```python
from build123d import *

# Parameters (mm, degrees)
PAD002_DEPTH   = 40
SKETCH006_R    = 1.5
HOLE_DEPTH     = 4.5
HOLE_TIPS_R    = 1.5
SKETCH002_R    = 1.5
HOLE001_DEPTH  = 4.5
HOLE001_TIPS_R = 1.5
SKETCH007_R    = 11
PAD003_DEPTH   = 2
PAD004_DEPTH   = 23


with BuildPart() as part:
    # Sketch005 → Pad002 (new body)
    with BuildSketch(Plane.XY):
        Polygon((-17.614466, 21.15), (17.614466, 21.15), (21.15, 17.614466), (21.15, -17.614466), (17.614466, -21.15), (-17.614466, -21.15), (-21.15, -17.614466), (-21.15, 17.614466), align=None)
    extrude(amount=PAD002_DEPTH)

    # Sketch006 (on Face10 of Pad002) → Hole (cut)
    with BuildSketch(Plane.XY.offset(40)):
        with Locations((15.5, 15.5)):
            Circle(SKETCH006_R)
        with Locations((-15.5, 15.5)):
            Circle(SKETCH006_R)
        with Locations((-15.5, -15.5)):
            Circle(SKETCH006_R)
        with Locations((15.5, -15.5)):
            Circle(SKETCH006_R)
    extrude(amount=-HOLE_DEPTH, mode=Mode.SUBTRACT)

    # Hole tips → Hole tip 1 section 0
    with BuildSketch(Plane.XY.offset(35.5), mode=Mode.PRIVATE) as hole_tip_1_s0:
        with Locations((15.5, 15.5)):
            Circle(HOLE_TIPS_R)
    loft([hole_tip_1_s0.sketch, Vertex(15.5, 15.5, 34.598709)], mode=Mode.SUBTRACT)

    # Hole tips → Hole tip 2 section 0
    with BuildSketch(Plane.XY.offset(35.5), mode=Mode.PRIVATE) as hole_tip_2_s0:
        with Locations((-15.5, 15.5)):
            Circle(HOLE_TIPS_R)
    loft([hole_tip_2_s0.sketch, Vertex(-15.5, 15.5, 34.598709)], mode=Mode.SUBTRACT)

    # Hole tips → Hole tip 3 section 0
    with BuildSketch(Plane.XY.offset(35.5), mode=Mode.PRIVATE) as hole_tip_3_s0:
        with Locations((-15.5, -15.5)):
            Circle(HOLE_TIPS_R)
    loft([hole_tip_3_s0.sketch, Vertex(-15.5, -15.5, 34.598709)], mode=Mode.SUBTRACT)

    # Hole tips → Hole tip 4 section 0
    with BuildSketch(Plane.XY.offset(35.5), mode=Mode.PRIVATE) as hole_tip_4_s0:
        with Locations((15.5, -15.5)):
            Circle(HOLE_TIPS_R)
    loft([hole_tip_4_s0.sketch, Vertex(15.5, -15.5, 34.598709)], mode=Mode.SUBTRACT)

    # Sketch002 → Hole001 (cut)
    with BuildSketch(Plane.XY):
        with Locations((-15.5, 15.5)):
            Circle(SKETCH002_R)
        with Locations((-15.5, -15.5)):
            Circle(SKETCH002_R)
        with Locations((15.5, -15.5)):
            Circle(SKETCH002_R)
        with Locations((15.5, 15.5)):
            Circle(SKETCH002_R)
    extrude(amount=HOLE001_DEPTH, mode=Mode.SUBTRACT)

    # Hole001 tips → Hole001 tip 1 section 0
    with BuildSketch(Plane.XY.offset(4.5), mode=Mode.PRIVATE) as hole001_tip_1_s0:
        with Locations((-15.5, 15.5)):
            Circle(HOLE001_TIPS_R)
    loft([hole001_tip_1_s0.sketch, Vertex(-15.5, 15.5, 5.401291)], mode=Mode.SUBTRACT)

    # Hole001 tips → Hole001 tip 2 section 0
    with BuildSketch(Plane.XY.offset(4.5), mode=Mode.PRIVATE) as hole001_tip_2_s0:
        with Locations((-15.5, -15.5)):
            Circle(HOLE001_TIPS_R)
    loft([hole001_tip_2_s0.sketch, Vertex(-15.5, -15.5, 5.401291)], mode=Mode.SUBTRACT)

    # Hole001 tips → Hole001 tip 3 section 0
    with BuildSketch(Plane.XY.offset(4.5), mode=Mode.PRIVATE) as hole001_tip_3_s0:
        with Locations((15.5, -15.5)):
            Circle(HOLE001_TIPS_R)
    loft([hole001_tip_3_s0.sketch, Vertex(15.5, -15.5, 5.401291)], mode=Mode.SUBTRACT)

    # Hole001 tips → Hole001 tip 4 section 0
    with BuildSketch(Plane.XY.offset(4.5), mode=Mode.PRIVATE) as hole001_tip_4_s0:
        with Locations((15.5, 15.5)):
            Circle(HOLE001_TIPS_R)
    loft([hole001_tip_4_s0.sketch, Vertex(15.5, 15.5, 5.401291)], mode=Mode.SUBTRACT)

    # Sketch007 (on Face5 of Hole001) → Pad003 (join)
    with BuildSketch(Plane.XY.offset(40)):
        Circle(SKETCH007_R)
    extrude(amount=PAD003_DEPTH)

    # Sketch008 (on Face27 of Pad003) → Pad004 (join)
    with BuildSketch(Plane.XY.offset(42)):
        with BuildLine():
            ThreePointArc((-1.581929, 1.6), (0, -2.25), (1.581929, 1.6))
            Line((-1.581929, 1.6), (1.581929, 1.6))
        make_face()
    extrude(amount=PAD004_DEPTH)


with BuildPart() as part_1:
    # Body001 placement: moved
    add(part.part.moved(Location((0, 0, -40))))


solid = part_1.part
```
Build history of the part. All positions in model axes, mm. A direction names the side the tool comes from. Round coordinates to 2 decimals unless told otherwise and drop trailing zeros. Loops run counter-clockwise (first coordinate to the right, second up) from the corner with the lowest first, then second, coordinate; pieces in that order, holes last.
Item 1: Saw through at A-A (z = -3.5). List the corners of the cut face in (x, y), then the cut area to 3 significant figures.
Item 2: Saw through at C-C (y = -4). List the corners of the cut face in (x, z), then the cut area to 3 significant figures.
Item 3: Drill centre lines: line 1 along Y through (x, z) = (-15.5, -37.4); line 2 along X through (y, z) = (-15, -1). Where is each one in solid material? Low to high.
Item 4: Saw through at B-B (x = 0). List the corners of the cut face in (y, z), then the cut area to 3 significant figures.
Item 5: Which spindle directions (+Z, -Z, +X, -X, +Y, -Y) get a long thin tool onto all of the face, cutting with end or side? Do faces 1 (the face through (-17, 15.57, -37.78)), 2 (the face through (-2.38, -10.74, 0.99)), 3 (the face through (0, 0, 25)). Say none if no direction does.
Item 6: Two-plate mould, pull along X, no slides. Class faces 4 (the face through (19.357, 19.407, -20.28)), 5 (the face through (-17, -15.43, -37.78)), 6 (the face through (0, 0, -40)), 7 (the face through (-17, 15.57, -2.22)): released by +X, released by -X, zero draft, split by the parting line, or undercut.
Item 7: Saw through at D-D (z = 19). List the corners of the cut face in (x, y).
Item 8: Pin check, flat tips, straight feed: P1, Ø5, axis at x = 8, y = 2.5, coming from the +Z side; P2, Ø4, axis at x = -15.5, y = 15.5, coming from the +Z side; P3, Ø1.8, axis at x = 15.5, y = -15.5, coming from the +Z side. Stop position of each tip, or through.
Worked answers:
1. outline: (-21.15, -17.61) - (-17.61, -21.15) - (17.61, -21.15) - (21.15, -17.61) - (21.15, 17.61) - (17.61, 21.15) - (-17.61, 21.15) - (-21.15, 17.61) - close; hole circle Ø3 at (-15.5, -15.5); hole circle Ø3 at (-15.5, 15.5); hole circle Ø3 at (15.5, -15.5); hole circle Ø3 at (15.5, 15.5)
1. area: 1,740 mm2
2. outline: (-21.15, -40) - (21.15, -40) - (21.15, 0) - (10.25, 0) - (10.25, 2) - (-10.25, 2) - (-10.25, 0) - (-21.15, 0) - close
2. area: 1,730 mm2
3. line 1: y = -21.15 to -17, -14 to 14, 17 to 21.15
3. line 2: x = -21.15 to -16.91, -14.09 to 14.09, 16.91 to 21.15
4. outline: (-21.15, -40) - (21.15, -40) - (21.15, 0) - (11, 0) - (11, 2) - (1.6, 2) - (1.6, 25) - (-2.25, 25) - (-2.25, 2) - (-11, 2) - (-11, 0) - (-21.15, 0) - close
4. area: 1,820 mm2
5. face 1: -Z
5. face 2: +Z
5. face 3: +Z, +X, -X, +Y, -Y
6. face 4: released by +X
6. face 5: undercut
6. face 6: zero draft
6. face 7: undercut
7. outline: (-1.58, 1.6) arc R2.25 ccw (long way) to (1.58, 1.6) - close
8. P1: stops at z = 2
8. P2: stops at z = 0
8. P3: stops at z = -4.86
